Geometry: final body of the model. Coordinates: model frame, mm. Face numbers are marked on the shaded views. A direction names the side the tool comes from. Coordinates: 2 decimals unless noted, no trailing zeros. Loops run counter-clockwise (first coordinate to the right, second up) from the corner with the lowest first, then second, coordinate; pieces in that order, holes last. Notation, with made-up numbers: M 78,-8 L 109,-8 A12 ccw 109,2 Z; hole C 15.5,65.25 d3. An arc over 180 degrees is marked long. Write each question's results on one line, items separated by ' | '. Start each with the question number.
from build123d import *

# Parameters (mm, degrees)
SKETCH1_W           = 57.15
SKETCH1_H           = 16.383
SKETCH1_R           = 3.175
BOSS_EXTRUDE1_DEPTH = 25.4
SKETCH1_4_W         = 57.15
SKETCH1_4_H         = 16.383
SKETCH1_4_R         = 3.175
CUT_EXTRUDE1_DEPTH  = 22.225
FILLET2_R           = 1.27
FILLET3_R           = 0.254


with BuildPart() as part:
    # Sketch1 → Boss-Extrude1 (new body, symmetric)
    with BuildSketch(Plane.XY):
        Rectangle(SKETCH1_W, SKETCH1_H)
        with Locations((-9.525, -1.8415)):
            Circle(SKETCH1_R, mode=Mode.SUBTRACT)
        with BuildLine():
            Line((28.575, 8.1915), (28.575, 11.3665))
            Line((28.575, 11.3665), (-9.525, 11.3665))
            ThreePointArc((-9.525, 11.3665), (-13.050132349, 9.650975764), (-16.910848847, 10.332481161))
            Line((-16.910848847, 10.332481161), (-28.575, 8.6995))
            Line((-28.575, 8.6995), (-28.575, 8.1915))
            Line((-28.575, 8.1915), (28.575, 8.1915))
        make_face()
        Polygon((28.575, 11.3665), (-9.525, 20.8915), (-9.525, 11.3665), align=None)
    extrude(amount=BOSS_EXTRUDE1_DEPTH, both=True)

    # Sketch1_4 → Cut-Extrude1 (cut, symmetric)
    with BuildSketch(Plane.XY):
        Rectangle(SKETCH1_4_W, SKETCH1_4_H)
        with Locations((-9.525, -1.8415)):
            Circle(SKETCH1_4_R, mode=Mode.SUBTRACT)
    extrude(amount=CUT_EXTRUDE1_DEPTH, both=True, mode=Mode.SUBTRACT)

    # Fillet2
    fillet2_edges = [part.edges().sort_by_distance(p)[0] for p in [
        (-28.575, -8.1915, 23.8125),
        (-16.910848847, 10.332481161, 0),
        (-9.525, 11.3665, 0),
        (-9.525, 20.8915, 0),
        (28.575, 11.3665, 0),
        (28.575, -8.1915, 23.8125),
        (-28.575, -8.1915, -23.8125),
        (28.575, -8.1915, -23.8125),
        (28.575, 8.1915, 0),
    ]]
    fillet(fillet2_edges, radius=FILLET2_R)

    # Fillet3
    fillet3_edges = [part.edges().sort_by_distance(p)[0] for p in [
        (-28.575, 8.6995, 0),
        (-28.575, 8.1915, 0),
    ]]
    fillet(fillet3_edges, radius=FILLET3_R)


solid = part.part
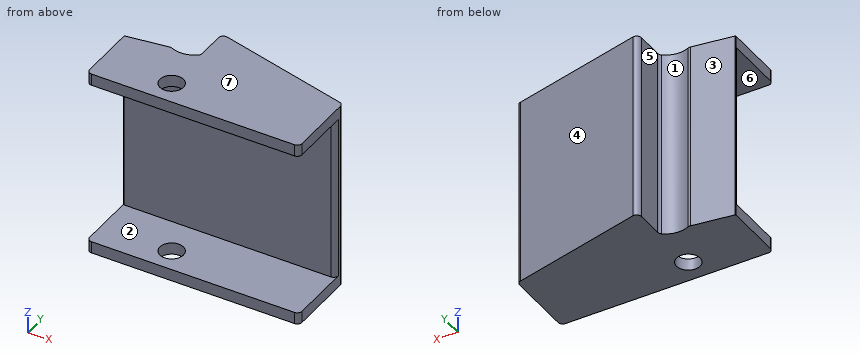
Item 1: Section A-A, the plane y = 6.5. Return loops of the section in (x, z) (3 decimals), plus the area to 3 significant figures.
Item 2: Section D-D, the plane y = -0.5. Return loops of the section in (x, z) (3 decimals).
Item 3: Contact query for flat-ended pins moving along their axis: P1, Ø6, axis at y = 17, z = -11, coming from the -X side (3 decimals); P2, Ø6, axis at x = -22, z = 10.5, coming from the +Y side; P3, Ø1, axis at x = 22, z = 10, coming from the +Y side. Output: stop coordinate, or through.
Item 4: Set-up query: the marked faces 5, 6 and 7. Return all of +Z, -Z, +X, -X, +Y, -Y with unobstructed straight access to the full face (end or side cutting, diameter ignored); none if empty.
Item 5: Pull-direction query (X, two-part tool) for the marked faces 1, 2, 3 and 4; classes: released by +X, released by -X, zero draft, split by the parting line, or undercut.
Item 6: Ray query, L1, parallel to Z at x = -18.5, y = 6.75 (3 decimals); L2, parallel to Y at x = 20.5, z = 6.5; L3, parallel to Y at x = -14.5, z = -23. Return the intervals inside material, ascending. Write a range as [from, to].
Solutions:
1) outline: M -28.575,-25.4 L 28.575,-25.4 L 28.575,-22.225 L -28.575,-22.225 Z; M -28.575,22.225 L 28.575,22.225 L 28.575,25.4 L -28.575,25.4 Z | area: 363 mm²
2) outline: M -28.575,-25.4 L -12.403,-25.4 L -12.403,-22.225 L -28.575,-22.225 Z; M -28.575,22.225 L -12.403,22.225 L -12.403,25.4 L -28.575,25.4 Z; M -6.647,-25.4 L 28.575,-25.4 L 28.575,-22.225 L -6.647,-22.225 Z; M -6.647,22.225 L 28.575,22.225 L 28.575,25.4 L -6.647,25.4 Z
3) P1: stops at x = -9.525 | P2: stops at y = 10.04 | P3: stops at y = 13.14
4) face 5: +Z, -Z, -X, +Y | face 6: +X, -X, -Y | face 7: +Z, +X, -X, +Y, -Y
5) face 1: undercut | face 2: zero draft | face 3: released by -X | face 4: released by +X
6) L1: z = [-25.4, -22.225], [22.225, 25.4] | L2: y = [8.19, 13.39] | L3: y = [-8.19, 9.62]
